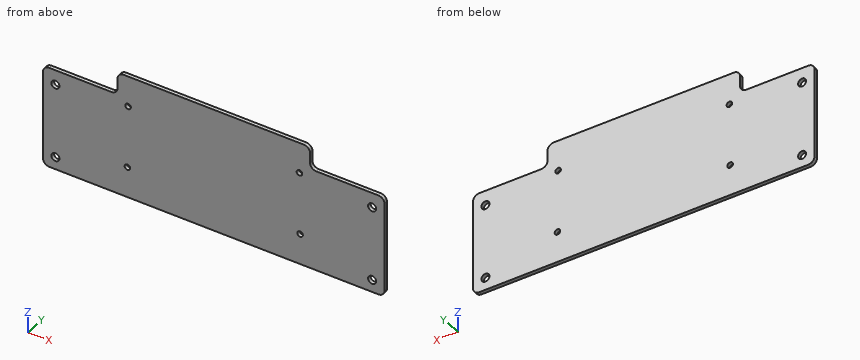
from build123d import *

# Parameters (mm, degrees)
F0_R     = 3.25
F0_R_2   = 2.25
F1_DEPTH = 3


with BuildPart() as f1:
    # F0 (on Front) → F1 (new body)
    with BuildSketch(Plane.XZ):
        with BuildLine():
            Line((-132.5, -50), (132.5, -50))
            ThreePointArc((132.5, -50), (136.035534, -48.535534), (137.5, -45))
            Line((137.5, -45), (137.5, 26.887341))
            ThreePointArc((137.5, 26.887341), (136.035534, 30.422875), (132.5, 31.887341))
            Line((132.5, 31.887341), (82.5, 31.887341))
            ThreePointArc((82.5, 31.887341), (78.964466, 33.351807), (77.5, 36.887341))
            Line((77.5, 36.887341), (77.5, 45))
            ThreePointArc((77.5, 45), (76.035534, 48.535534), (72.5, 50))
            Line((72.5, 50), (-72.5, 50))
            ThreePointArc((-72.5, 50), (-76.035534, 48.535534), (-77.5, 45))
            Line((-77.5, 45), (-77.5, 36.887341))
            ThreePointArc((-77.5, 36.887341), (-78.964466, 33.351807), (-82.5, 31.887341))
            Line((-82.5, 31.887341), (-132.5, 31.887341))
            ThreePointArc((-132.5, 31.887341), (-136.035534, 30.422875), (-137.5, 26.887341))
            Line((-137.5, 26.887341), (-137.5, -45))
            ThreePointArc((-137.5, -45), (-136.035534, -48.535534), (-132.5, -50))
        make_face()
        with Locations((-127.5, -40)):
            Circle(F0_R, mode=Mode.SUBTRACT)
        with Locations((-69.5, -25.25)):
            Circle(F0_R_2, mode=Mode.SUBTRACT)
        with Locations((127.5, -40)):
            Circle(F0_R, mode=Mode.SUBTRACT)
        with Locations((69.5, -25.25)):
            Circle(F0_R_2, mode=Mode.SUBTRACT)
        with Locations((-127.5, 20)):
            Circle(F0_R, mode=Mode.SUBTRACT)
        with BuildLine():
            ThreePointArc((-69, 27.5), (-67.40901, 26.84099), (-66.75, 25.25))
            ThreePointArc((-66.75, 25.25), (-67.40901, 23.65901), (-69, 23))
            ThreePointArc((-69, 23), (-71.25, 25.25), (-69, 27.5))
        make_face(mode=Mode.SUBTRACT)
        with Locations((127.5, 20)):
            Circle(F0_R, mode=Mode.SUBTRACT)
        with Locations((69, 25.25)):
            Circle(F0_R_2, mode=Mode.SUBTRACT)
    extrude(amount=F1_DEPTH)


solid = f1.part
Verification items for the finished model (mm, model axes). Coordinates: 2 decimals unless noted, no trailing zeros. Order: outer loops, then holes, each group sorted by start corner. A loop starts at its lowest first (then second) coordinate and runs counter-clockwise, first axis right, second up. Notation, with made-up numbers: M -18.5,11 L 16.5,11 A28 cw 16.5,34 Z; hole C 37.25,22.25 d1. An arc over 180 degrees is marked long. One line per item, written item: value. Start each with the question number.
Item 1: Sectioned sample at C-C (y = -0.55). Count the separate pieces of the cut face and the enclosed holes in it, then the cut area to 3 significant figures.
Item 2: Sectioned sample at D-D (x = 94.5). Enter the section's corners in (y, z).
Item 3: Scan lines: probe 1 along Z at (x, y) = (-127.5, -1); probe 2 along Z at (x, y) = (69.5, -1.8); probe 3 along X at (y, z) = (-1.25, 27). Record each from-to range of solid material in increasing order.
Item 4: Gauge pin test, flat ends, axial feed: pin 1 (0.9 mm diameter, centred on x = -115, y = -2, fed in from +Z); pin 2 (1.5 mm diameter, centred on y = -1, z = 40.5, fed in from -X); pin 3 (1.5 mm diameter, centred on y = -2, z = 40.5, fed in from +X). Record the tip position at first contact, or that the pin passes through.
Item 5: Sectioned sample at A-A (x = -127.5). Enter the section's corners in (y, z).
Item 6: Sectioned sample at B-B (z = 20). Enter the section's corners in (x, y).
Conclusion:
1. separate pieces: 1
1. enclosed holes: 8
1. area: 25,100 mm^2
2. outline: M -3,-50 L 0,-50 L 0,31.89 L -3,31.89 Z
3. probe 1: z = -50 to -43.25, -36.75 to 16.75, 23.25 to 31.89
3. probe 2: z = -50 to -27.5, -23 to 23.06, 27.44 to 50
3. probe 3: x = -137.5 to -70.41, -67.59 to 67.59, 70.41 to 137.5
4. pin 1: stops at z = 31.89
4. pin 2: stops at x = -77.5
4. pin 3: stops at x = 77.5
5. outline: M -3,-50 L 0,-50 L 0,-43.25 L -3,-43.25 Z; M -3,-36.75 L 0,-36.75 L 0,16.75 L -3,16.75 Z; M -3,23.25 L 0,23.25 L 0,31.89 L -3,31.89 Z
6. outline: M -137.5,-3 L -130.75,-3 L -130.75,0 L -137.5,0 Z; M -124.25,-3 L 124.25,-3 L 124.25,0 L -124.25,0 Z; M 130.75,-3 L 137.5,-3 L 137.5,0 L 130.75,0 Z
